The model under review builds one solid part; all positions refer to its coordinate system, in mm. Face numbers are marked on the shaded views. A direction names the side the tool comes from. Coordinates: 2 decimals unless noted, no trailing zeros. Order: outer loops, then holes, each group sorted by start corner. A loop starts at its lowest first (then second) coordinate and runs counter-clockwise, first axis right, second up. Notation, with made-up numbers: (49.25, 76) -> (83.25, 76) arc R33 cw to (83.25, 106) -> close; hole circle Ø5 at (28.25, -36.75). An arc over 180 degrees is marked (long way). Put each result on its own line as item: value.
from build123d import *

# Parameters (mm, degrees)
EXTRUDE_4_DEPTH     = 2
EXTRUDE_5_DEPTH     = 12
EXTRUDE_START       = -12
EXTRUDE_7_DEPTH     = 1
CUT_EXTRUDE_START   = 2
CUT_EXTRUDE_4_DEPTH = 11
CUT_EXTRUDE_5_REACH = 119.533
SKETCH_4_W          = 10
SKETCH_4_H          = 5


with BuildPart() as part:
    # Эскиз1 → Бобышка-Вытянуть4 (new body)
    with BuildSketch(Plane(origin=(0, 0, 0), x_dir=(1, 0, 0), z_dir=(0, 1, 0))):
        with BuildLine():
            Line((-2.084374602, -1.449446306), (-2.084374602, -72.949446306))
            ThreePointArc((-2.084374602, -72.949446306), (-0.619908508, -76.484980212), (2.915625398, -77.949446306))
            Line((2.915625398, -77.949446306), (79.915625398, -77.949446306))
            ThreePointArc((79.915625398, -77.949446306), (83.451159304, -76.484980212), (84.915625398, -72.949446306))
            Line((84.915625398, -72.949446306), (84.915625398, -1.449446306))
            ThreePointArc((84.915625398, -1.449446306), (83.451159304, 2.0860876), (79.915625398, 3.550553694))
            Line((79.915625398, 3.550553694), (2.915625398, 3.550553694))
            ThreePointArc((2.915625398, 3.550553694), (-0.619908508, 2.0860876), (-2.084374602, -1.449446306))
        make_face()
    extrude(amount=EXTRUDE_4_DEPTH)

    # Эскиз1<9> → Бобышка-Вытянуть5 (add)
    with BuildSketch(Plane(origin=(0, 0, 0), x_dir=(1, 0, 0), z_dir=(0, 1, 0))):
        with BuildLine():
            Line((-2.084374602, -1.449446306), (-2.084374602, -72.949446306))
            ThreePointArc((-2.084374602, -72.949446306), (-0.619908508, -76.484980212), (2.915625398, -77.949446306))
            Line((2.915625398, -77.949446306), (79.915625398, -77.949446306))
            ThreePointArc((79.915625398, -77.949446306), (83.451159304, -76.484980212), (84.915625398, -72.949446306))
            Line((84.915625398, -72.949446306), (84.915625398, -1.449446306))
            ThreePointArc((84.915625398, -1.449446306), (83.451159304, 2.0860876), (79.915625398, 3.550553694))
            Line((79.915625398, 3.550553694), (2.915625398, 3.550553694))
            ThreePointArc((2.915625398, 3.550553694), (-0.619908508, 2.0860876), (-2.084374602, -1.449446306))
        make_face()
        with BuildLine():
            Line((-0.084374602, -1.449446306), (-0.084374602, -72.949446306))
            ThreePointArc((-0.084374602, -72.949446306), (0.794305055, -75.070766649), (2.915625398, -75.949446306))
            Line((2.915625398, -75.949446306), (79.915625398, -75.949446306))
            ThreePointArc((79.915625398, -75.949446306), (82.036945742, -75.070766649), (82.915625398, -72.949446306))
            Line((82.915625398, -72.949446306), (82.915625398, -1.449446306))
            ThreePointArc((82.915625398, -1.449446306), (82.036945742, 0.671874038), (79.915625398, 1.550553694))
            Line((79.915625398, 1.550553694), (2.915625398, 1.550553694))
            ThreePointArc((2.915625398, 1.550553694), (0.794305055, 0.671874038), (-0.084374602, -1.449446306))
        make_face(mode=Mode.SUBTRACT)
    extrude(amount=EXTRUDE_5_DEPTH)

    # Эскиз3 → Бобышка-Вытянуть7 (add)
    with BuildSketch(Plane.XZ.offset(EXTRUDE_START)):
        with BuildLine():
            Line((2.915625398, -2.550553694), (79.915625398, -2.550553694))
            ThreePointArc((79.915625398, -2.550553694), (82.744052523, -1.378980819), (83.915625398, 1.449446306))
            Line((83.915625398, 1.449446306), (83.915625398, 72.949446306))
            ThreePointArc((83.915625398, 72.949446306), (82.744052523, 75.777873431), (79.915625398, 76.949446306))
            Line((79.915625398, 76.949446306), (2.915625398, 76.949446306))
            ThreePointArc((2.915625398, 76.949446306), (0.087198273, 75.777873431), (-1.084374602, 72.949446306))
            Line((-1.084374602, 72.949446306), (-1.084374602, 1.449446306))
            ThreePointArc((-1.084374602, 1.449446306), (0.087198273, -1.378980819), (2.915625398, -2.550553694))
        make_face()
    extrude(amount=-EXTRUDE_7_DEPTH)

    # Эскиз1<13> → Вырез-Вытянуть4 (cut)
    with BuildSketch(Plane(origin=(0, 0, 0), x_dir=(1, 0, 0), z_dir=(0, 1, 0)).offset(CUT_EXTRUDE_START)):
        with BuildLine():
            Line((-0.084374602, -1.449446306), (-0.084374602, -72.949446306))
            ThreePointArc((-0.084374602, -72.949446306), (0.794305055, -75.070766649), (2.915625398, -75.949446306))
            Line((2.915625398, -75.949446306), (79.915625398, -75.949446306))
            ThreePointArc((79.915625398, -75.949446306), (82.036945742, -75.070766649), (82.915625398, -72.949446306))
            Line((82.915625398, -72.949446306), (82.915625398, -1.449446306))
            ThreePointArc((82.915625398, -1.449446306), (82.036945742, 0.671874038), (79.915625398, 1.550553694))
            Line((79.915625398, 1.550553694), (2.915625398, 1.550553694))
            ThreePointArc((2.915625398, 1.550553694), (0.794305055, 0.671874038), (-0.084374602, -1.449446306))
        make_face()
    extrude(amount=CUT_EXTRUDE_4_DEPTH, mode=Mode.SUBTRACT)

    # Эскиз4 → Вырез-Вытянуть5 (cut, up to next)
    with BuildSketch(Plane(origin=(84.915625398, 0, 0), x_dir=(0, 0, -1), z_dir=(1, 0, 0)), mode=Mode.PRIVATE) as cut_extrude_5_sk1:
        with Locations((-9.449446306, 12.5)):
            Rectangle(SKETCH_4_W, SKETCH_4_H)
    cut_extrude_5_tool1 = extrude(cut_extrude_5_sk1.sketch, amount=-CUT_EXTRUDE_5_REACH, mode=Mode.PRIVATE) & part.part
    add(cut_extrude_5_tool1.solids().sort_by_distance((84.915625, 12.5, 9.449446))[0], mode=Mode.SUBTRACT)


solid = part.part
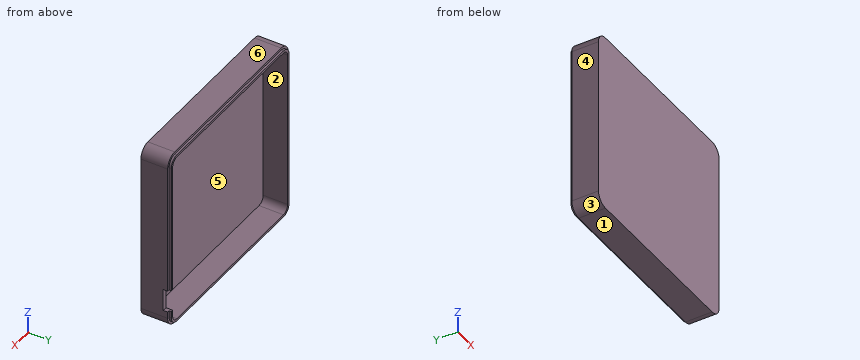
Item 1: For the marked faces 1 and 2, list the 3-axis set-ups (+Z, -Z, +X, -X, +Y, -Y) from which the entire face can be reached by the end or side of a thin tool; tool diameter is ignored.
Answers below:
face 1: -Z, +X, -X, +Y, -Y
face 2: +Y
Item 2: For pin 1 Ø0.5 at (y, z) = (12.5, 39) entering from +X; pin 2 Ø8 at (x, z) = (46.5, 39) entering from +Y; pin 3 Ø1 at (x, y) = (83.5, 12) entering from +Z, all flat-tipped, find the tip position at first contact; note any pin that passes through.
Answers below:
pin 1: x = 83.92
pin 2: y = 2
pin 3: z = 76.88
Item 3: Mouldability with a two-part tool opening along Z and no side actions: class the marked faces 3, 4, 5 and 6 as +Z half, -Z half, draft (parallel to the pull), parting line (faces both ways), or undercut.
Answers below:
face 3: -Z half
face 4: draft
face 5: undercut
face 6: +Z half
Item 4: For line 1 (X direction, y = 2.75, z = 9.5); line 2 (Z direction, x = 13, y = 2.5); line 3 (X direction, y = 12.25, z = 21), list the stretches that pass through material, from the lowest coordinate up. Write a range as from..to.
Answers below:
line 1: -2.08..-0.08, 82.92..84.92
line 2: -3.55..-1.55, 75.95..77.95
line 3: -1.08..-0.08, 82.92..83.92
Item 5: Consider section A-A on x = 5. Write out the cut boundary in (y, z).
Answers below:
outline: (0, -3.55) -> (12, -3.55) -> (12, -2.55) -> (13, -2.55) -> (13, -1.55) -> (2, -1.55) -> (2, 75.95) -> (13, 75.95) -> (13, 76.95) -> (12, 76.95) -> (12, 77.95) -> (0, 77.95) -> close
Item 6: Consider section B-B on y = 5. Write out the cut boundary in (x, z).
Answers below:
outline: (-2.08, 1.45) arc R5 ccw to (2.92, -3.55) -> (79.92, -3.55) arc R5 ccw to (84.92, 1.45) -> (84.92, 72.95) arc R5 ccw to (79.92, 77.95) -> (2.92, 77.95) arc R5 ccw to (-2.08, 72.95) -> close; hole (-0.08, 1.45) arc R3 ccw to (2.92, -1.55) -> (79.92, -1.55) arc R3 ccw to (82.92, 1.45) -> (82.92, 72.95) arc R3 ccw to (79.92, 75.95) -> (2.92, 75.95) arc R3 ccw to (-0.08, 72.95) -> close
Item 7: Consider section D-D on y = 11. Write out the cut boundary in (x, z).
Answers below:
outline: (-2.08, 1.45) arc R5 ccw to (2.92, -3.55) -> (79.92, -3.55) arc R5 ccw to (84.92, 1.45) -> (84.92, 4.45) -> (82.92, 4.45) -> (82.92, 1.45) arc R3 cw to (79.92, -1.55) -> (2.92, -1.55) arc R3 cw to (-0.08, 1.45) -> (-0.08, 72.95) arc R3 cw to (2.92, 75.95) -> (79.92, 75.95) arc R3 cw to (82.92, 72.95) -> (82.92, 14.45) -> (84.92, 14.45) -> (84.92, 72.95) arc R5 ccw to (79.92, 77.95) -> (2.92, 77.95) arc R5 ccw to (-2.08, 72.95) -> close
Item 8: Consider section C-C on z = 69. Write out the cut boundary in (x, y).
Answers below:
outline: (-2.08, 0) -> (84.92, 0) -> (84.92, 12) -> (83.92, 12) -> (83.92, 13) -> (82.92, 13) -> (82.92, 2) -> (-0.08, 2) -> (-0.08, 13) -> (-1.08, 13) -> (-1.08, 12) -> (-2.08, 12) -> close
